Geometry: final body of the model. Coordinates: model frame, mm. A direction names the side the tool comes from. Round coordinates to 2 decimals unless told otherwise and drop trailing zeros. Write each loop counter-clockwise with the first axis right and the second up, starting at its lowest first coordinate (ties: lowest second). Pieces come first, ordered by that corner, then holes. Notation, with made-up numbers: M 46,82 L 86,82 A6 ccw 86,89 Z; hole C 84.25,66 d3. An arc over 180 degrees is marked long. Put each result on its own line as item: value. Start each with the question number.
```python
from build123d import *

# Parameters (mm, degrees)
SKETCH1_W                                       = 85.999999704
SKETCH1_H                                       = 99.314
BOSS_EXTRUDE1_DEPTH                             = 63.903125051
SKETCH2_W                                       = 75.999999892
SKETCH2_H                                       = 68.834
CUT_EXTRUDE1_DEPTH                              = 92.642932229
F_6_5_6_5_DIAMETER_HOLE1_D                      = 6.5
F_6_5_6_5_DIAMETER_HOLE1_DEPTH                  = 4.999999906
F_12_0_12_DIAMETER_HOLE1_D                      = 12
F_12_0_12_DIAMETER_HOLE1_DEPTH                  = 4.999999906
CSK_FOR_M3_FLAT_HEAD_MACHINE_SCREW1_D           = 3.4
CSK_FOR_M3_FLAT_HEAD_MACHINE_SCREW1_DEPTH       = 4.999999906
CSK_FOR_M3_FLAT_HEAD_MACHINE_SCREW1_CSINK_D     = 6.3
CSK_FOR_M3_FLAT_HEAD_MACHINE_SCREW1_CSINK_ANGLE = 90
F_10_CLEARANCE_HOLE1_D                          = 5.1054
SKETCH12_R                                      = 6.499999954
CUT_EXTRUDE2_DEPTH                              = 2.499999953


with BuildPart() as part:
    # Sketch1 → Boss-Extrude1 (new body)
    with BuildSketch(Plane.XY):
        Rectangle(SKETCH1_W, SKETCH1_H)
    extrude(amount=BOSS_EXTRUDE1_DEPTH)

    # Sketch2 → Cut-Extrude1 (cut, through all)
    with BuildSketch(Plane.XY.offset(63.903125051)):
        Rectangle(SKETCH2_W, SKETCH2_H)
    extrude(amount=-CUT_EXTRUDE1_DEPTH, mode=Mode.SUBTRACT)

    # Ø6.5 (6.5) Diameter Hole1
    with Locations(Plane(origin=(42.999999852, 0, 0), x_dir=(0, 0, -1), z_dir=(1, 0, 0))):
        with Locations((-14.450199954, -9.525)):
            Hole(F_6_5_6_5_DIAMETER_HOLE1_D / 2, depth=F_6_5_6_5_DIAMETER_HOLE1_DEPTH)

    # Ø12.0 (12) Diameter Hole1
    with Locations(Plane.ZY.offset(42.999999852)):
        with Locations((45.403125094, -15.917000043)):
            Hole(F_12_0_12_DIAMETER_HOLE1_D / 2, depth=F_12_0_12_DIAMETER_HOLE1_DEPTH)

    # CSK for M3 Flat Head Machine Screw1
    with Locations(Plane.ZY.offset(42.999999852)):
        with Locations((45.403125094, -0.417000055), (58.826518842, -8.167000049), (58.826518842, -23.667000037), (45.403125094, -31.417000031), (31.979731346, -23.667000037), (31.979731346, -8.167000049)):
            CounterSinkHole(CSK_FOR_M3_FLAT_HEAD_MACHINE_SCREW1_D / 2, CSK_FOR_M3_FLAT_HEAD_MACHINE_SCREW1_CSINK_D / 2, depth=CSK_FOR_M3_FLAT_HEAD_MACHINE_SCREW1_DEPTH, counter_sink_angle=CSK_FOR_M3_FLAT_HEAD_MACHINE_SCREW1_CSINK_ANGLE)

    # #10 Clearance Hole1 (through all)
    with Locations(Plane.XY.offset(63.903125051)):
        with Locations((-35.379999852, 42.037), (35.379999852, 42.037), (-35.379999852, -42.037), (35.379999852, -42.037)):
            Hole(F_10_CLEARANCE_HOLE1_D / 2)

    # Sketch12 → Cut-Extrude2 (cut)
    with BuildSketch(Plane(origin=(42.999999852, 0, 0), x_dir=(0, 0, -1), z_dir=(1, 0, 0))):
        with Locations((-14.450199954, -9.525)):
            Circle(SKETCH12_R)
    extrude(amount=-CUT_EXTRUDE2_DEPTH, mode=Mode.SUBTRACT)


solid = part.part
```
1) Draft query along Y for faces 5 (the face through (43, -1, 32)), 6 (the face through (38, 0, 32)), 7 (the face through (-1, -49.657, 32)). Return one class per face: +Y half, -Y half, draft (parallel to the pull), parting line (faces both ways), or undercut.
2) Access query for faces 1 (the face through (-3, -37, 0)), 2 (the face through (41.77, -13.48, 19.61)), 3 (the face through (-1, 34.417, 32)), 4 (the face through (-39.75, -7.656, 57.205)). Directions: +Z, -Z, +X, -X, +Y, -Y. A direction counts if a zero-diameter tool reaches every point of the face in a straight line with its end or side. Return the directions, or none.
3) Section A-A, the plane x = 19. Output: boundary loops of the cut face in (y, z).
4) Section B-B, the plane y = 14. Output: boundary loops of the cut face in (x, z).
5) Section D-D, the plane z = 26.5. Output: boundary loops of the cut face in (x, y).
6) Section C-C, the plane x = -35.38. Output: boundary loops of the cut face in (y, z), and give its area (3 significant figures).
7) First-contact query: pin 1 (2.5 mm diameter, centred on y = -8.17, z = 31.98, fed in from -X); pin 2 (3 mm diameter, centred on x = -35.38, y = 42.037, fed in from +Z); pin 3 (4 mm diameter, centred on y = -23.67, z = 31.98, fed in from -X); pin 4 (5.5 mm diameter, centred on y = -8.17, z = 58.83, fed in from -X). Flat tips, straight axial feed; report the tip coordinate or a pass-through.
8) Ray query, probe 1 along Y at (x, z) = (21, 56.5); probe 2 along X at (y, z) = (21, 48.5); probe 3 along Y at (x, z) = (-35.5, 59). Return the intervals inside material, ascending.
Solved:
1. face 5: draft
1. face 6: undercut
1. face 7: -Y half
2. face 1: -Z, +X, -X, +Y, -Y
2. face 2: +X
2. face 3: +Z, -Z
2. face 4: -X
3. outline: M -49.66,0 L -34.42,0 L -34.42,63.9 L -49.66,63.9 Z; M 34.42,0 L 49.66,0 L 49.66,63.9 L 34.42,63.9 Z
4. outline: M -43,0 L -38,0 L -38,63.9 L -43,63.9 Z; M 38,0 L 43,0 L 43,63.9 L 38,63.9 Z
5. outline: M -43,-49.66 L 43,-49.66 L 43,49.66 L -43,49.66 Z; hole M -38,-34.42 L 38,-34.42 L 38,34.42 L -38,34.42 Z; hole C -35.38,-42.04 d5.11; hole C -35.38,42.04 d5.11; hole C 35.38,-42.04 d5.11; hole C 35.38,42.04 d5.11
6. outline: M -49.66,0 L -44.59,0 L -44.59,63.9 L -49.66,63.9 Z; M -39.48,0 L -34.42,0 L -34.42,63.9 L -39.48,63.9 Z; M 34.42,0 L 39.48,0 L 39.48,63.9 L 34.42,63.9 Z; M 44.59,0 L 49.66,0 L 49.66,63.9 L 44.59,63.9 Z
6. area: 1,300 mm2
7. pin 1: stops at x = 38
7. pin 2: passes through
7. pin 3: stops at x = -41.85
7. pin 4: stops at x = -42.6
8. probe 1: y = -49.66 to -34.42, 34.42 to 49.66
8. probe 2: x = -43 to -38, 38 to 43
8. probe 3: y = -49.66 to -44.59, -39.49 to -34.42, 34.42 to 39.49, 44.59 to 49.66
